from build123d import *

# Parameters (mm, degrees)
F2_R     = 1.75
F3_DEPTH = 1.001


# Not quite as in the source:
# - a fillet or chamfer that OpenCascade refuses, or shapes differently, is made with other operations: its cross-section is extruded or revolved along the edge and cut away or added


with BuildPart() as f1:
    # F0 (on Front) → F1 (revolve)
    with BuildSketch(Plane.XZ):
        Polygon((0, 1), (0, 0), (9, 0), (5, 5), (4, 5), (4, 1), align=None)
    revolve(axis=Axis((0, 0, 2.5), (0, 0, 1)))

    # F2 (on face) → F3 (cut, through all)
    with BuildSketch(Plane.XY.offset(1)):
        Circle(F2_R)
    extrude(amount=-F3_DEPTH, mode=Mode.SUBTRACT)

    # F4: fillet of radius 5 on 1 edges, made by hand

    # F4_s1 → F4_t2 (revolve, cut)
    with BuildSketch(Plane.XZ):
        with BuildLine():
            ThreePointArc((6.2858644818, 3.3926693977), (5.2575025417, 4.3592707998), (4, 5))
            Line((4, 5), (5, 5))
            Line((5, 5), (6.2858644818, 3.3926693977))
        make_face()
    revolve(axis=Axis((0, 0, 5), (0, 0, 1)), mode=Mode.SUBTRACT)


solid = f1.part
Build history of the part. All positions in model axes, mm. Round coordinates to 2 decimals unless told otherwise and drop trailing zeros. Write each loop counter-clockwise with the first axis right and the second up, starting at its lowest first coordinate (ties: lowest second). Pieces come first, ordered by that corner, then holes. Notation, with made-up numbers: M 63,6 L 97,6 A26 cw 97,25 Z; hole C -8,37 d6. An arc over 180 degrees is marked long. Answer as a JSON object with one key per item and string values. Group by question number.
(1) Flat gauge pins, fed straight in: pin 1 (3 mm diameter, centred on y = 0.5, z = 3.5, fed in from +X); pin 2 (1 mm diameter, centred on y = -4, z = 3.5, fed in from +X); pin 3 (3 mm diameter, centred on y = 1.5, z = 0.5, fed in from +X). Where does each tip first touch, or does it go through?
(2) Mould opens along Y. For faces 1 (the flat face through (0, -2, 0)), 2 (the conical face through (3, -5.7, 3.2)), 3 (the flat face through (2, -1, 1)), 4 (the cylindrical face through (-0.867, -3.905, 2.972)) say: pulls with the +Y half, pulls with the -Y half, needs draft (parallel to the pull), parting line crosses it, or undercut.
(3) Drill centre lines: L1, parallel to Z at x = 1.75, y = 3; L2, parallel to Y at x = 0.5, z = 1.45; L3, parallel to Y at x = 1.25, z = 0.35. Where is each one in solid material? Low to high.
(4) Cut at A-A (z = 0.65). Give the cut face in (x, y), and give its area (3 significant figures).
Responses:
{
 "1": {"pin 1": "stops at x = 7.39", "pin 2": "stops at x = 5.37", "pin 3": "stops at x = 9"},
 "2": {"face 1": "needs draft", "face 2": "parting line crosses it", "face 3": "undercut", "face 4": "undercut"},
 "3": {"L1": "z = 0 to 1", "L2": "y = -7.82 to -3.97, 3.97 to 7.82", "L3": "y = -8.63 to -1.22, 1.22 to 8.63"},
 "4": {"outline": "C 0,0 d16.96; hole C 0,0 d3.5", "area": "216 mm2"}
}
